Check sheet for the drawn part. Datum: minimum x, y, z corner. Units: mm. A direction names the side the tool comes from. Give positions to 0.01 mm unless a question says otherwise; leave off trailing zeros. Loops run counter-clockwise (first coordinate to the right, second up) from the corner with the lowest first, then second, coordinate; pieces in that order, holes last. Notation, with made-up numbers: (-8, 73) - (26, 73) arc R38 ccw to (26, 112) - close; hole circle Ø2 at (-38.75, 19.5). An arc over 180 degrees is marked (long way). Use one line per item in the form item = value.
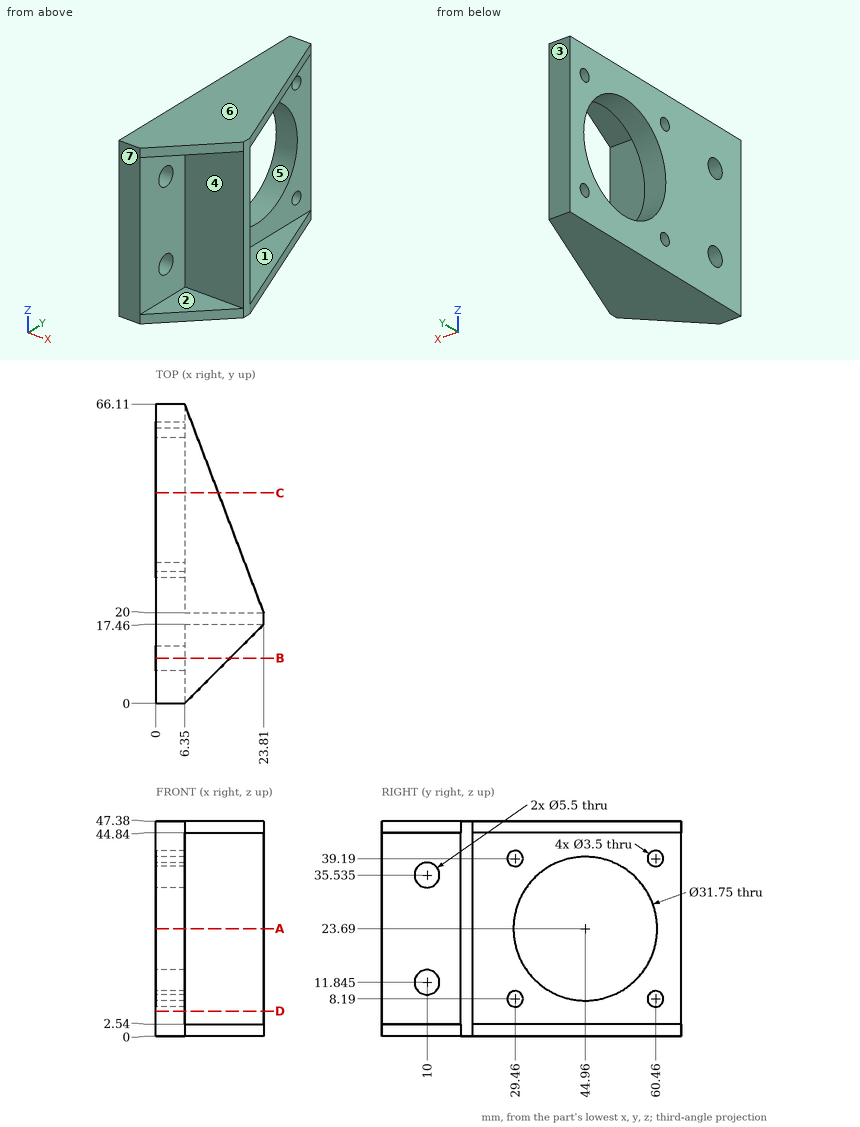
Item 1: Access from +Z, -Z, +X, -X, +Y, -Y to the whole of each face (thin tool, end or side, straight path). Record for the marked faces 1, 2 and 3.
Answer block:
face_1 = +X, +Y
face_2 = +X, -Y
face_3 = +Z, -Z, +X, -X, +Y
Item 2: Thickness scan on L1, parallel to Z at x = 5, y = 10 (3 decimals); L2, parallel to Z at x = 4, y = 44.96 (3 decimals); L3, parallel to Z at x = 10.5, y = 37. Record the ranges inside material, lowest first.
Answer block:
L1 = 0 to 9.095, 14.595 to 32.785, 38.285 to 47.38
L2 = 0 to 7.815, 39.565 to 47.38
L3 = 0 to 2.54, 44.84 to 47.38
Item 3: Section check B-B on y = 10. Record the boundary of the cut face in (x, z) (3 decimals), then the cut area to 3 significant figures.
Answer block:
outline = (0, 0) - (16.35, 0) - (16.35, 2.54) - (6.35, 2.54) - (6.35, 9.095) - (0, 9.095) - close; (0, 14.595) - (6.35, 14.595) - (6.35, 32.785) - (0, 32.785) - close; (0, 38.285) - (6.35, 38.285) - (6.35, 44.84) - (16.35, 44.84) - (16.35, 47.38) - (0, 47.38) - close
area = 282 mm2
Item 4: Mould release check, pull along Z, two halves, no side actions. Record for the marked faces 4, 5, 6 and 7: released by +Z, released by -Z, zero draft, split by the parting line, or undercut.
Answer block:
face_4 = undercut
face_5 = undercut
face_6 = released by +Z
face_7 = zero draft
Item 5: Gauge pin test, flat ends, axial feed: P1, Ø14, axis at x = 18, z = 14, coming from the -Y side; P2, Ø4.5, axis at y = 10, z = 11.845, coming from the +X side; P3, Ø12.5, axis at y = 53, z = 30, coming from the +X side; P4, Ø8.5, axis at x = 17, z = 16.5, coming from the +Y side. Record the tip position at first contact, or that the pin passes through.
Answer block:
P1 = 17.46
P2 = through
P3 = 6.35
P4 = 20
Item 6: Section check D-D on z = 5.5. Record the boundary of the cut face in (x, y), then the cut area to 3 significant figures.
Answer block:
outline = (0, 0) - (6.35, 0) - (6.35, 17.46) - (23.81, 17.46) - (23.81, 20) - (6.35, 20) - (6.35, 66.11) - (0, 66.11) - close
area = 464 mm2
Item 7: Section check A-A on z = 23.69. Record the boundary of the cut face in (x, y) (3 decimals).
Answer block:
outline = (0, 0) - (6.35, 0) - (6.35, 17.46) - (23.81, 17.46) - (23.81, 20) - (6.35, 20) - (6.35, 29.085) - (0, 29.085) - close; (0, 60.835) - (6.35, 60.835) - (6.35, 66.11) - (0, 66.11) - close
Item 8: Section check C-C on y = 46.5. Record the boundary of the cut face in (x, z).
Answer block:
outline = (0, 0) - (13.78, 0) - (13.78, 2.54) - (6.35, 2.54) - (6.35, 7.89) - (0, 7.89) - close; (0, 39.49) - (6.35, 39.49) - (6.35, 44.84) - (13.78, 44.84) - (13.78, 47.38) - (0, 47.38) - close
